Answer from the drawing. Dimensions are ordinates in mm from the lowest x, y and z of the part. Round coordinates to 2 decimals unless told otherwise and drop trailing zeros. Loops run counter-clockwise (first coordinate to the right, second up) from the corner with the lowest first, then second, coordinate; pieces in that order, holes last. Notation, with made-up numbers: (60, -31.75) - (90, -31.75) arc R15 cw to (90, -26.75) - close; hole circle Ø9 at (55.5, 73). An arc over 180 degrees is marked (long way). Answer as CSV lines item,"result". Start each with the question number.
Q1. Section C-C on z = 11 is taken. Write down the section's boundary in (x, y) (3 decimals).
Q2. Straight lines are drawn through the part: L1, parallel to X at y = 38.1, z = 7.5 (3 decimals); L2, parallel to Y at x = 38.1, z = 6. For each, find the intervals that lie inside material, in ascending order. Write a range as [from, to].
Q3. Each of these flat-tipped pins is pushed along its axis until it touches: pin 1 Ø3 at (y, z) = (62, 16.5) entering from -X; pin 2 Ø3 at (x, z) = (18.5, 18) entering from -Y; pin 3 Ø1 at (x, z) = (50.5, 10) entering from -Y. Where does it stop, or does it pass through?
Q4. Section A-A on x = 38.1 is taken. Write down the section's boundary in (y, z) (3 decimals).
Q5. The mould has two halves that part along X. Classify the marked faces 1, 2 and 3: +X half, -X half, draft (parallel to the pull), parting line (faces both ways), or undercut.
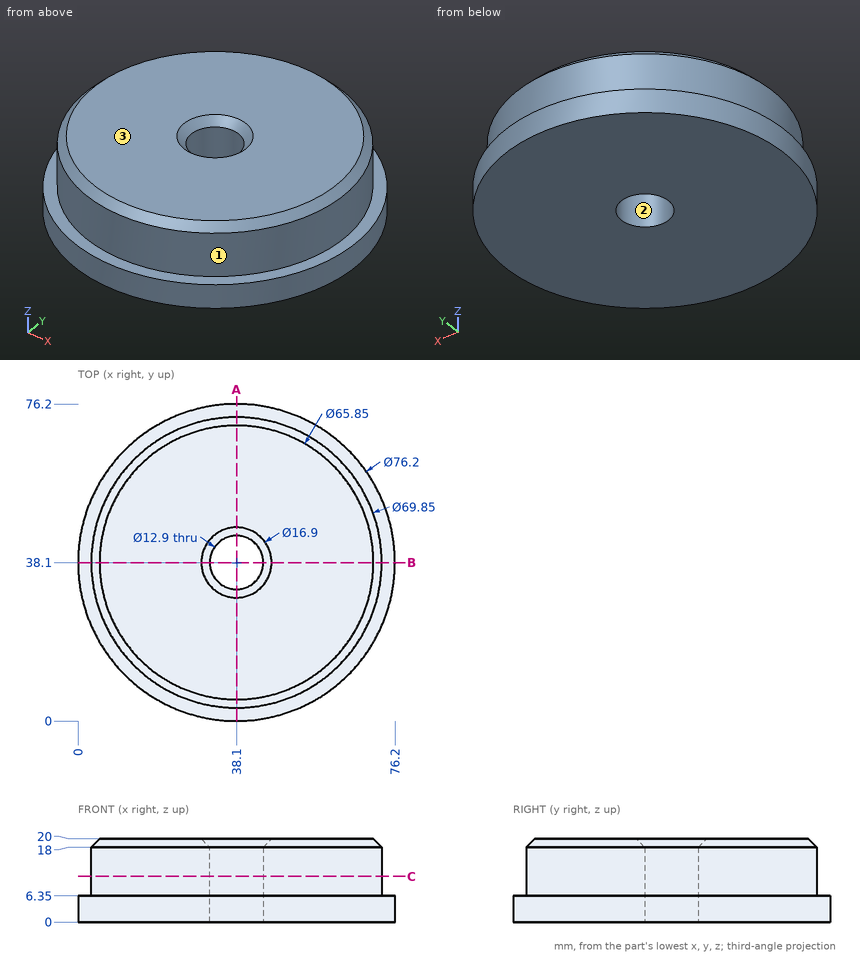
Findings:
1,outline,"circle Ø69.85 at (38.1, 38.1); hole circle Ø12.9 at (38.1, 38.1)"
2,L1,"x = [3.175, 31.65], [44.55, 73.025]"
2,L2,"y = [0, 31.65], [44.55, 76.2]"
3,pin 1,"stops at x = 11.3"
3,pin 2,"stops at y = 8.23"
3,pin 3,"stops at y = 5.26"
4,outline,"(0, 0) - (31.65, 0) - (31.65, 18) - (29.65, 20) - (5.175, 20) - (3.175, 18) - (3.175, 6.35) - (0, 6.35) - close; (44.55, 0) - (76.2, 0) - (76.2, 6.35) - (73.025, 6.35) - (73.025, 18) - (71.025, 20) - (46.55, 20) - (44.55, 18) - close"
5,face 1,"parting line"
5,face 2,"undercut"
5,face 3,"draft"
